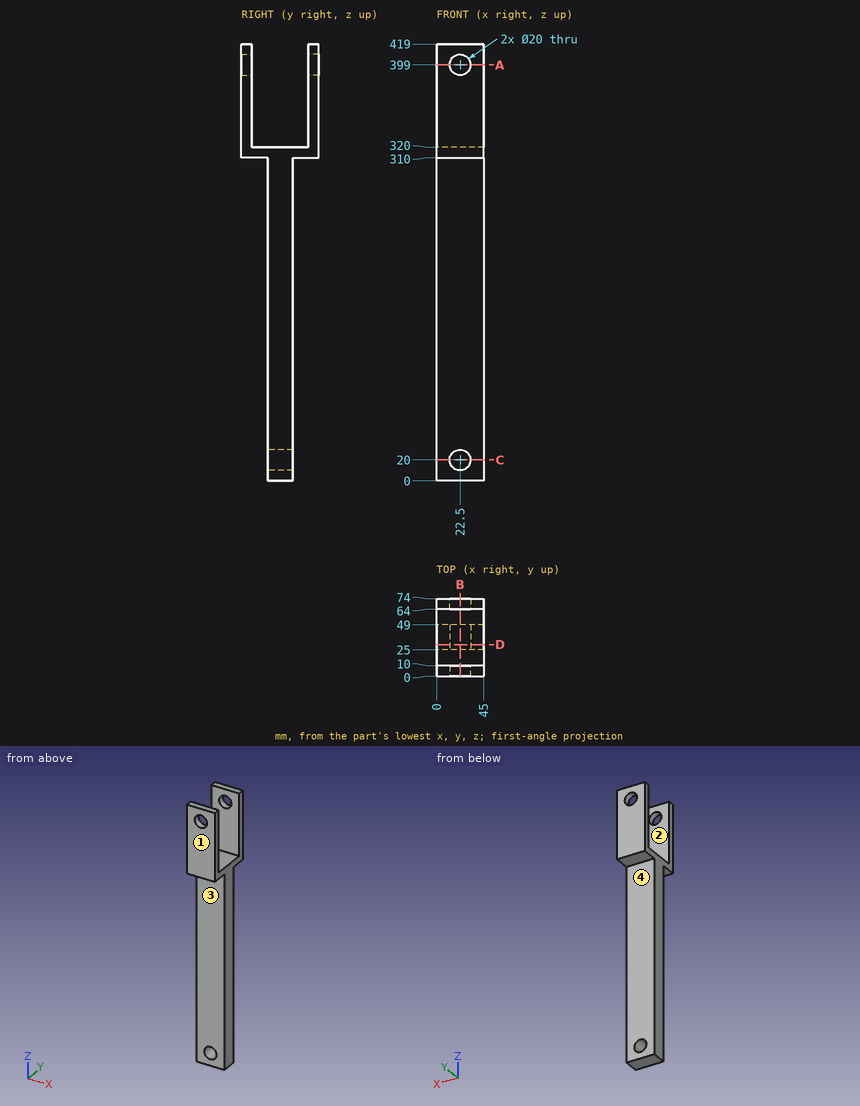
Check sheet for the drawn part. Datum: minimum x, y, z corner. Units: mm. A direction names the side the tool comes from. Give positions to 0.01 mm unless a question says otherwise; leave off trailing zeros. Loops run counter-clockwise (first coordinate to the right, second up) from the corner with the lowest first, then second, coordinate; pieces in that order, holes last. Notation, with made-up numbers: M 37.5,35 L 61.5,35 A23 cw 61.5,53 Z; hole C -5,51.5 d3. An arc over 180 degrees is marked long. Answer as CSV lines item,"result".
Item 1: Depth check by flat-ended pin: pin 1 Ø13.5 at (x, y) = (27.5, 38) entering from +Z; pin 2 Ø13.5 at (x, z) = (27, 376) entering from -Y; pin 3 Ø10 at (x, z) = (31, 288) entering from -Y; pin 4 Ø2 at (x, z) = (30, 98) entering from +Y. Enter the tip coordinate at first touch or a pass-through.
Reply:
pin 1,"z = 320"
pin 2,"y = 0"
pin 3,"y = 25"
pin 4,"y = 49"
Item 2: Set-up check for the marked faces 1, 2, 3 and 4: record each of +Z, -Z, +X, -X, +Y, -Y from which the full face is reachable in a straight line by a thin tool's end or side.
Reply:
face 1,"+Z, -Z, +X, -X, -Y"
face 2,"+Z, +X, -X"
face 3,"-Z, +X, -X, -Y"
face 4,"-Z, +X, -X, +Y"
Item 3: Sectioned sample at D-D, the plane y = 30. Enter the section's corners in (x, z), then the cut area to 3 significant figures.
Reply:
outline,"M 0,0 L 45,0 L 45,320 L 0,320 Z; hole C 22.5,20 d20"
area,"14,100 mm^2"
Item 4: Sectioned sample at B-B, the plane x = 22.5. Enter the section's corners in (y, z), then the cut area to 3 significant figures.
Reply:
outline,"M 0,310 L 25,310 L 25,30 L 49,30 L 49,310 L 74,310 L 74,389 L 64,389 L 64,320 L 10,320 L 10,389 L 0,389 Z; M 0,409 L 10,409 L 10,419 L 0,419 Z; M 25,0 L 49,0 L 49,10 L 25,10 Z; M 64,409 L 74,409 L 74,419 L 64,419 Z"
area,"9,280 mm^2"
Item 5: Sectioned sample at A-A, the plane z = 399. Enter the section's corners in (x, y), then the cut area to 3 significant figures.
Reply:
outline,"M 0,0 L 12.5,0 L 12.5,10 L 0,10 Z; M 0,64 L 12.5,64 L 12.5,74 L 0,74 Z; M 32.5,0 L 45,0 L 45,10 L 32.5,10 Z; M 32.5,64 L 45,64 L 45,74 L 32.5,74 Z"
area,"500 mm^2"
Item 6: Sectioned sample at C-C, the plane z = 20. Enter the section's corners in (x, y).
Reply:
outline,"M 0,25 L 12.5,25 L 12.5,49 L 0,49 Z; M 32.5,25 L 45,25 L 45,49 L 32.5,49 Z"
Item 7: Scan lines: L1, parallel to X at y = 36, z = 20; L2, parallel to Y at x = 4.5, z = 330; L3, parallel to Z at x = 22, y = 7. Record each from-to range of solid material in increasing order.
Reply:
L1,"0 to 12.5, 32.5 to 45"
L2,"0 to 10, 64 to 74"
L3,"310 to 389.01, 408.99 to 419"
